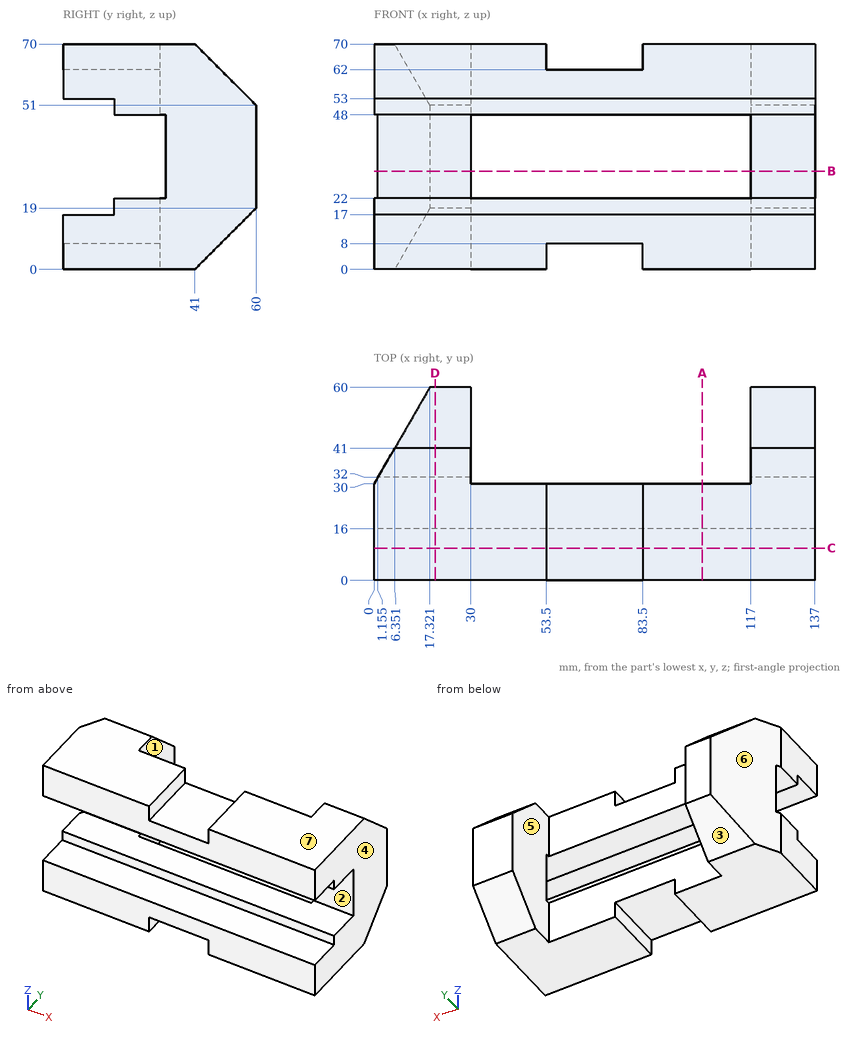
Input: dimensioned drawing with shaded views. Units: mm. Origin: part minimum x, y, z. A direction names the side the tool comes from. Give positions to 0.01 mm unless a question says otherwise; leave off trailing zeros. Loops run counter-clockwise (first coordinate to the right, second up) from the corner with the lowest first, then second, coordinate; pieces in that order, holes last. Notation, with made-up numbers: (60, 52) -> (96, 52) arc R20 ccw to (96, 56) -> close; hole circle Ø8 at (68.25, 8.5). An arc over 180 degrees is marked (long way). Use a Markdown table: item, result. Add a question column.
1) Pull-direction query (X, two-part tool) for the marked faces 4, 5, 6 and 7; classes: +X half, -X half, draft (parallel to the pull), parting line (faces both ways), or undercut.
2) First-contact query: pin 1 (1.5 mm diameter, centred on x = 77.5, y = 11.5, fed in from +Z); pin 2 (2.5 mm diameter, centred on x = 101, z = 18.5, fed in from -Y); pin 3 (24 mm diameter, centred on x = 90, z = 64, fed in from +Y); pin 4 (17.5 mm diameter, centred on x = 40.5, y = 11.5, fed in from -Z). Flat tips, straight axial feed; report the tip coordinate or a pass-through.
3) Line query: line 1 along Z through (x, y) = (103, 25); line 2 along Z through (x, y) = (119.5, 10); line 3 along X through (y, z) = (14.5, 5). Output: solid intervals per line, ascending. Write a range as [from, to].
4) Section query C-C, the plane y = 10. Return the cut outline in (x, z), then the cut area to 3 significant figures.
5) Reachability of the marked faces 1, 2 and 3 from +Z, -Z, +X, -X, +Y, -Y: full face, straight path, thin tool, end or side. Return the list, or none.
6) Section query B-B, the plane z = 30.5. Return the cut outline in (x, y) (1 decimal).
7) Section query D-D, the plane x = 19. Return the cut outline in (y, z).
8) Section query A-A, the plane x = 102. Return the cut outline in (y, z), then the cut area to 3 significant figures.
Numbers:
| question | item | result |
|---|---|---|
| 1 | face 4 | +X half |
| 1 | face 5 | undercut |
| 1 | face 6 | -X half |
| 1 | face 7 | draft |
| 2 | pin 1 | stops at z = 62 |
| 2 | pin 2 | stops at y = 16 |
| 2 | pin 3 | stops at y = 30 |
| 2 | pin 4 | stops at z = 0 |
| 3 | line 1 | z = [0, 22], [48, 70] |
| 3 | line 2 | z = [0, 17], [53, 70] |
| 3 | line 3 | x = [0, 53.5], [83.5, 137] |
| 4 | outline | (0, 0) -> (53.5, 0) -> (53.5, 8) -> (83.5, 8) -> (83.5, 0) -> (137, 0) -> (137, 17) -> (0, 17) -> close; (0, 53) -> (137, 53) -> (137, 70) -> (83.5, 70) -> (83.5, 62) -> (53.5, 62) -> (53.5, 70) -> (0, 70) -> close |
| 4 | area | 4,180 mm2 |
| 5 | face 1 | +Z, -Z, +Y |
| 5 | face 2 | +X, -X, -Y |
| 5 | face 3 | -Z, +X, -X, +Y |
| 6 | outline | (1.2, 32) -> (30, 32) -> (30, 60) -> (17.3, 60) -> close; (117, 32) -> (137, 32) -> (137, 60) -> (117, 60) -> close |
| 7 | outline | (0, 0) -> (41, 0) -> (60, 19) -> (60, 51) -> (41, 70) -> (0, 70) -> (0, 53) -> (16, 53) -> (16, 48) -> (32, 48) -> (32, 22) -> (16, 22) -> (16, 17) -> (0, 17) -> close |
| 8 | outline | (0, 0) -> (30, 0) -> (30, 22) -> (16, 22) -> (16, 17) -> (0, 17) -> close; (0, 53) -> (16, 53) -> (16, 48) -> (30, 48) -> (30, 70) -> (0, 70) -> close |
| 8 | area | 1,160 mm2 |
